For this review, use the dimensioned drawing (mm, ordinates from the lowest corner) and the shaded views. A direction names the side the tool comes from. Coordinates: 2 decimals unless noted, no trailing zeros. Order: outer loops, then holes, each group sorted by start corner. A loop starts at its lowest first (then second) coordinate and runs counter-clockwise, first axis right, second up. Notation, with made-up numbers: M 11.5,31 L 67.5,31 A32 cw 67.5,63 Z; hole C -40,-22.75 d2. An arc over 180 degrees is marked long. Write each question's results on one line, items separated by ' | '.
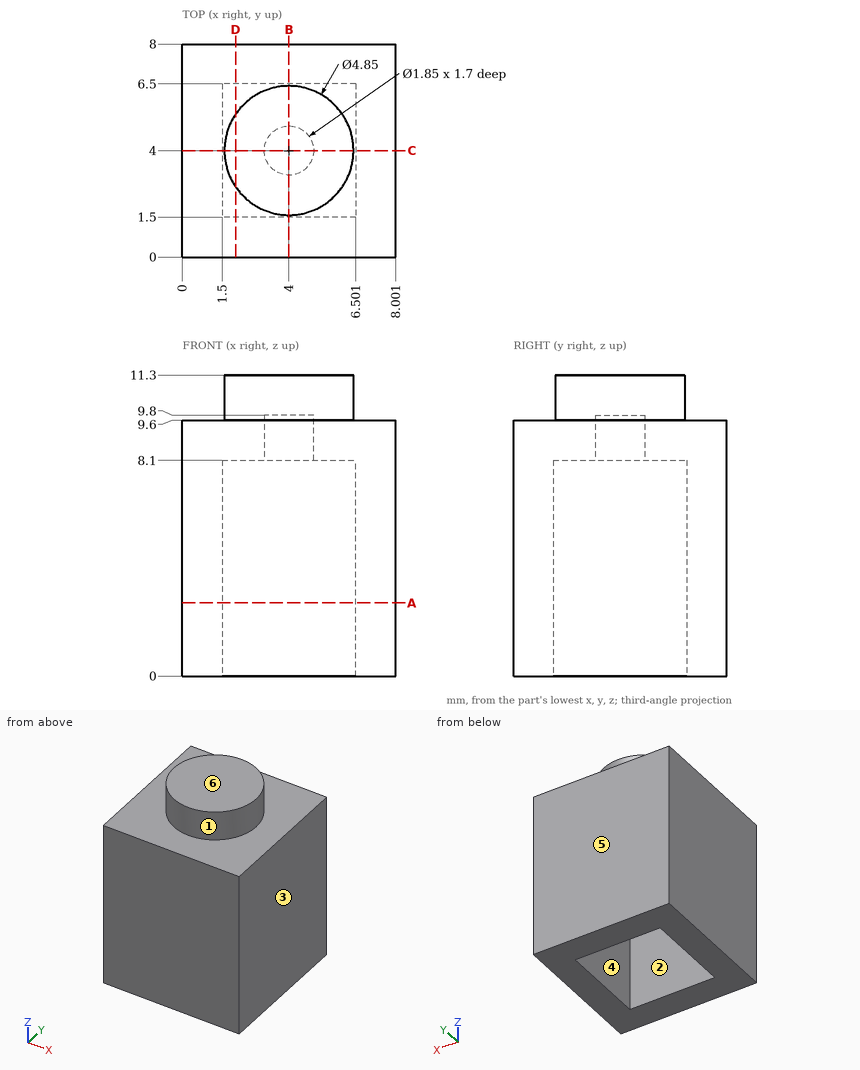
1) For the marked faces 1, 2 and 3, list the 3-axis set-ups (+Z, -Z, +X, -X, +Y, -Y) from which the entire face can be reached by the end or side of a thin tool; tool diameter is ignored.
Solutions:
face 1: +Z | face 2: -Z | face 3: +Z, -Z, +X, +Y, -Y
2) Take a section at D-D on x = 2. State the section outline as (y, z) points.
Solutions:
outline: M 0,0 L 1.5,0 L 1.5,8.1 L 6.5,8.1 L 6.5,0 L 8,0 L 8,9.6 L 5.37,9.6 L 5.37,11.3 L 2.63,11.3 L 2.63,9.6 L 0,9.6 Z
3) For pin 1 (1.5 mm diameter, centred on x = 4.5, y = 4.5, fed in from -Z), flat-tipped, find the tip position at first contact; note if it passes through.
Solutions:
pin 1: z = 8.1
4) Take a section at A-A on z = 2.75. State the section outline as (x, y) points.
Solutions:
outline: M 0,0 L 8,0 L 8,8 L 0,8 Z; hole M 1.5,1.5 L 6.5,1.5 L 6.5,6.5 L 1.5,6.5 Z
5) The part is to be moulded in two halves that separate along Y. For the marked faces 4, 5 and 6, say which applies: pulls with the +Y half, pulls with the -Y half, needs draft (parallel to the pull), parting line crosses it, or undercut.
Solutions:
face 4: undercut | face 5: pulls with the +Y half | face 6: needs draft
6) Take a section at B-B on x = 4. State the section outline as (y, z) points (1 decimal).
Solutions:
outline: M 0,0 L 1.5,0 L 1.5,8.1 L 3.1,8.1 L 3.1,9.8 L 4.9,9.8 L 4.9,8.1 L 6.5,8.1 L 6.5,0 L 8,0 L 8,9.6 L 6.4,9.6 L 6.4,11.3 L 1.6,11.3 L 1.6,9.6 L 0,9.6 Z
7) To check wall thickness, follow line 1 along Y through (x, z) = (4.25, 5.5); line 2 along X through (y, z) = (4, 9.25) (1 decimal). State the ranges of each line that lie inside material, in increasing order.
Solutions:
line 1: 0 to 1.5, 6.5 to 8 | line 2: 0 to 3.1, 4.9 to 8
